The listing builds one solid part. Answer for the finished solid, in the listing's coordinates (mm). A direction names the side the tool comes from. Give positions to 0.01 mm unless a question says otherwise; leave off trailing zeros. Order: outer loops, then holes, each group sorted by start corner. A loop starts at its lowest first (then second) coordinate and runs counter-clockwise, first axis right, second up. Notation, with made-up numbers: (-36.5, 42) - (10.5, 42) arc R18 cw to (10.5, 66) - close; hole circle Ø2 at (-11.5, 22.5). An arc over 180 degrees is marked (long way). Answer as a JSON object with one key per item and string values. Group by question number.
Q1. Given pin 1 (1 mm diameter, centred on x = -22.5, z = 1, fed in from +Y); pin 2 (4 mm diameter, centred on x = -169.57, y = 105.61, fed in from +Z); pin 3 (1.5 mm diameter, centred on y = 21.5, z = 0, fed in from -X), each flat-ended and moving along its own axis, determine where each tip first touches the part or whether it passes through.
Q2. A cutting plane is placed at A-A, the plane y = 95. Give the vertices of the cut face in (x, z), and give its area (3 significant figures).
Q3. A cutting plane is placed at B-B, the plane x = -145. Give the vertices of the cut face in (y, z), and give its area (3 significant figures).
Q4. Consider line 1 (X direction, y = -1, z = -0.4); line 2 (X direction, y = 18.5, z = -1.4); line 3 (Y direction, x = -66, z = -0.3). Determine where each line is inside the solid, lowest interval first.
Q5. For faces 1 (the face through (-116, 28, -2.5)), 2 (the face through (-154.481, 29, 0)), determine the directions among +Z, -Z, +X, -X, +Y, -Y from which every point of the face is accessible in a straight line to the end or side of a thin tool.
from build123d import *

# Parameters (mm, degrees)
BOSS_EXTRUDE1_DEPTH = 2.5
SKETCH3_R           = 1.5875
CUT_EXTRUDE1_DEPTH  = 214.852130583


with BuildPart() as part:
    # Sketch1 → Boss-Extrude1 (new, symmetric)
    with BuildSketch(Plane.XY):
        with BuildLine():
            Line((-154.481439558, -6.35), (-154.481439558, 66.347378373))
            Line((-154.481439558, 66.347378373), (-177.895895312, 99.786686688))
            ThreePointArc((-177.895895312, 99.786686688), (-176.041196233, 113.449531488), (-162.274426085, 112.681888078))
            Line((-162.274426085, 112.681888078), (-138.606439558, 88.2396))
            add(Edge.make_bspline(
                [(-138.606439558, 88.2396), (-138.606439558, 88.206480064), (-138.604893224, 88.134332137), (-138.597757085, 87.982040168), (-138.584504009, 87.767973581), (-138.563362589, 87.511833211), (-138.514302662, 87.023426652), (-138.425196169, 86.336581908), (-138.262733573, 85.340165391), (-137.997774346, 84.039042844), (-137.543893872, 82.163940465), (-136.709143666, 79.332808223), (-135.381511976, 75.692405853), (-133.427089014, 71.311625777), (-130.978665346, 66.686011286), (-128.248792738, 62.200876138), (-125.278396767, 57.871801388), (-121.922980854, 53.47598485), (-117.499907722, 48.25477976), (-111.846477366, 42.372548658), (-104.806706424, 36.032698765), (-96.481239759, 29.625824358), (-87.711829988, 23.843138375), (-78.562226684, 18.684637722), (-69.088219119, 14.150320925), (-59.340712588, 10.240190432), (-49.365347684, 6.954244107), (-41.111501611, 4.791563651), (-34.694119901, 3.420549472), (-30.177735786, 2.597379945), (-27.586849558, 2.166008761), (-24.349433278, 1.675559443), (-20.435573897, 1.165043535), (-15.888225625, 0.68322541), (-11.278370624, 0.337947753), (-7.392012303, 0.139524343), (-4.35262006, 0.048647043), (-2.477110072, 0.012428268), (-0.93320285, 0.001817838), (-0.315317676, 0), (0, 0)],
                knots=[0, 0, 0, 0, 0, 0.000750682, 0.001501364, 0.003002728, 0.004504092, 0.006005456, 0.011632897, 0.017260339, 0.025307868, 0.033355398, 0.051377592, 0.078047856, 0.105080676, 0.132113154, 0.15914583, 0.186178382, 0.213211084, 0.24601624, 0.3000815, 0.354146872, 0.408211991, 0.462277325, 0.516342503, 0.570407831, 0.624473028, 0.67853828, 0.732603517, 0.746119838, 0.759636158, 0.773152478, 0.786668798, 0.813701417, 0.840734035, 0.867766658, 0.88128297, 0.894799281, 0.901946134, 0.909092986, 0.909092986, 0.909092986, 0.909092986, 0.909092986], degree=4))
            Line((0, 0), (0, -6.35))
            Line((0, -6.35), (-154.481439558, -6.35))
        make_face()
    extrude(amount=BOSS_EXTRUDE1_DEPTH, both=True)

    # Sketch3 → Cut-Extrude1 (cut, through all)
    with BuildSketch(Plane.XY.offset(2.5)):
        with Locations((-169.573310542, 105.614223281)):
            Circle(SKETCH3_R)
    extrude(amount=-CUT_EXTRUDE1_DEPTH, mode=Mode.SUBTRACT)


solid = part.part
Reply:
{
 "1": {"pin 1": "stops at y = 1.51", "pin 2": "stops at z = 2.5", "pin 3": "stops at x = -154.48"},
 "2": {"outline": "(-174.54, -2.5) - (-145.15, -2.5) - (-145.15, 2.5) - (-174.54, 2.5) - close", "area": "147 mm^2"},
 "3": {"outline": "(-6.35, -2.5) - (94.84, -2.5) - (94.84, 2.5) - (-6.35, 2.5) - close", "area": "506 mm^2"},
 "4": {"line 1": "x = -154.48 to 0", "line 2": "x = -154.48 to -77.89", "line 3": "y = -6.35 to 12.99"},
 "5": {"face 1": "-Z, +X, -X, +Y, -Y", "face 2": "+Z, -Z, -X, -Y"}
}
